Design review of the part built by this model. Coordinates are the model's own, in mm. Face numbers are marked on the shaded views. A direction names the side the tool comes from. Give positions to 0.01 mm unless a question says otherwise; leave off trailing zeros. Order: outer loops, then holes, each group sorted by start corner. A loop starts at its lowest first (then second) coordinate and runs counter-clockwise, first axis right, second up.
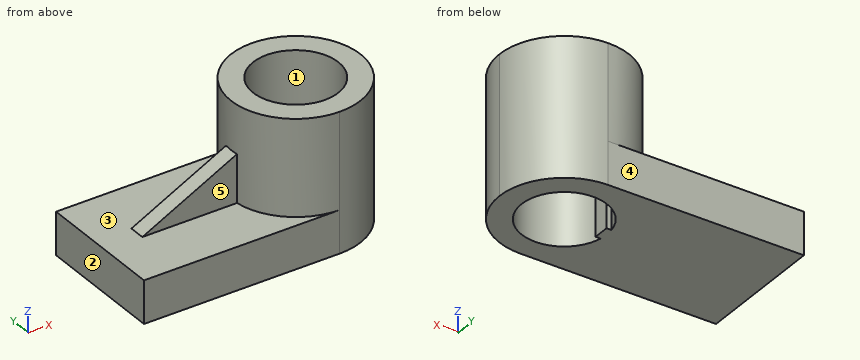
```python
from build123d import *

# Parameters (mm, degrees)
F0_R     = 25.404221
F1_DEPTH = 82.55
F2_DEPTH = 25.4
F3_W     = 72.80118
F3_H     = 9.580332
F4_DEPTH = 53.848
F6_DEPTH = 25.4


with BuildPart() as f1:
    # F0 (on Top) → F1 (new body)
    with BuildSketch(Plane.XY):
        with BuildLine():
            ThreePointArc((96.964516, 0), (85.654314, 27.305241), (58.349073, 38.615443))
            ThreePointArc((58.349073, 38.615443), (19.73363, 0), (58.349073, -38.615443))
            ThreePointArc((58.349073, -38.615443), (85.654314, -27.305241), (96.964516, 0))
        make_face()
        with Locations((58.349073, 0)):
            Circle(F0_R, mode=Mode.SUBTRACT)
    extrude(amount=F1_DEPTH)

    # F0 (on Top) → F2 (join)
    with BuildSketch(Plane.XY):
        with BuildLine():
            Line((58.349073, 38.615443), (-58.349073, 38.615443))
            Line((-58.349073, 38.615443), (-58.349073, -38.615443))
            Line((-58.349073, -38.615443), (58.349073, -38.615443))
            ThreePointArc((58.349073, -38.615443), (19.73363, 0), (58.349073, 38.615443))
        make_face()
    extrude(amount=F2_DEPTH)

    # F3 (on Top) → F4 (join)
    with BuildSketch(Plane.XY):
        Rectangle(F3_W, F3_H)
    extrude(amount=F4_DEPTH)

    # F5 (on face) → F6 (cut)
    with BuildSketch(Plane.XZ.offset(4.790166)):
        Polygon((-36.40059, 25.4), (20.031887, 53.848), (-36.40059, 53.848), align=None)
    extrude(amount=-F6_DEPTH, mode=Mode.SUBTRACT)


solid = f1.part
```
1. Take a section at C-C (x = -28.5). State the section outline as (y, z) points.
Recorded:
outline: (-38.62, 0) - (38.62, 0) - (38.62, 25.4) - (4.79, 25.4) - (4.79, 29.38) - (-4.79, 29.38) - (-4.79, 25.4) - (-38.62, 25.4) - close
2. For pin 1 (4 mm diameter, centred on x = 11, z = 40, fed in from +Y); pin 2 (14 mm diameter, centred on x = -16, z = 40, fed in from -Y); pin 3 (2 mm diameter, centred on y = -28, z = 48, fed in from +X), all flat-tipped, find the tip position at first contact; note any pin that passes through.
Recorded:
pin 1: stops at y = 4.79
pin 2: stops at y = -4.79
pin 3: stops at x = 85.96
3. Take a section at B-B (x = 54). State the section outline as (y, z) points, then the cut area to 3 significant figures.
Recorded:
outline: (-38.62, 0) - (-25.03, 0) - (-25.03, 82.55) - (-38.37, 82.55) - (-38.37, 25.4) - (-38.62, 25.4) - close; (25.03, 0) - (38.62, 0) - (38.62, 25.4) - (38.37, 25.4) - (38.37, 82.55) - (25.03, 82.55) - close
area: 2,220 mm2
4. Take a section at D-D (z = 28.5). State the section outline as (x, y) points, then the cut area to 3 significant figures.
Recorded:
outline: (-30.25, -4.79) - (20.03, -4.79) arc R38.62 ccw to (58.35, -38.62) arc R38.62 ccw to (96.96, 0) arc R38.62 ccw to (58.35, 38.62) arc R38.62 ccw to (20.03, 4.79) - (-30.25, 4.79) - close; hole (33.4, -4.79) arc R25.4 ccw (long way) to (33.4, 4.79) - (36.4, 4.79) - (36.4, -4.79) - close
area: 3,170 mm2
5. Draft analysis for pull direction X (two halves, no side actions). For the marked faces 1, 2 and 3, state which applies: pulls with the +X half, pulls with the -X half, needs draft (parallel to the pull), parting line crosses it, or undercut.
Recorded:
face 1: undercut
face 2: pulls with the -X half
face 3: needs draft
6. For line 1 along X through (y, z) = (0, 17); line 2 along Z through (x, y) = (27, 26); line 3 along Y through (x, z) = (72, 33), list the stretches that pass through material, from the lowest coordinate up.
Recorded:
line 1: x = -58.35 to 36.4, 83.75 to 96.96
line 2: z = 0 to 25.4
line 3: y = -36.12 to -21.42, 21.42 to 36.12
7. Machinability: for the marked faces 4 and 5, which of the approach directions +Z, -Z, +X, -X, +Y, -Y give a long, thin tool a straight path to every point of the face, cutting with its end or side? Answer none if there is none.
Recorded:
face 4: +Z, -Z, +X, -X, +Y
face 5: +Z, -X, -Y
8. Take a section at A-A (z = 7). State the section outline as (x, y) points.
Recorded:
outline: (-58.35, -38.62) - (58.35, -38.62) arc R38.62 ccw to (96.96, 0) arc R38.62 ccw to (58.35, 38.62) - (-58.35, 38.62) - close; hole (33.4, -4.79) arc R25.4 ccw (long way) to (33.4, 4.79) - (36.4, 4.79) - (36.4, -4.79) - close
